Geometry check sheet. Reference: the model listing, model coordinates, mm. Face numbers are marked on the shaded views. A direction names the side the tool comes from. Round coordinates to 2 decimals unless told otherwise and drop trailing zeros. Write each loop counter-clockwise with the first axis right and the second up, starting at its lowest first coordinate (ties: lowest second). Pieces come first, ordered by that corner, then holes. Notation, with made-up numbers: M -22,13 L 37,13 A35 cw 37,50 Z; hole C 72.25,-29.5 d8. An arc over 180 degrees is marked long. Put each result on its own line as item: value. Start each with the question number.
(1) Section check C-C on y = 12. Record the cut outline in (x, z).
(2) Material ranges on probe 1 along Y at (x, z) = (6.5, 0); probe 2 along Z at (x, y) = (6, 0); probe 3 along Y at (x, z) = (20, -26), recorded low to high.
(3) Gauge pin test, flat ends, axial feed: pin 1 (10 mm diameter, centred on x = -12.5, z = -13, fed in from -Y); pin 2 (8 mm diameter, centred on x = -10.27, y = 0, fed in from +Z); pin 3 (12 mm diameter, centred on x = 13.5, z = 7.5, fed in from -Y); pin 4 (8 mm diameter, centred on y = 17, z = -15.5, fed in from +X). Record the tip position at first contact, or that the pin passes through.
(4) Section check D-D on x = 3. Record the cut outline in (y, z).
(5) Section check A-A on x = 20. Record the cut outline in (y, z).
(6) Section check B-B on z = -12.5. Record the cut outline in (x, y).
(7) Tool access check on the marked faces 1, 2 and 3. Record the directions out of +Z, -Z, +X, -X, +Y, -Y that give a thin tool (end or side, any length) a straight path to the whole face; none if there is none.
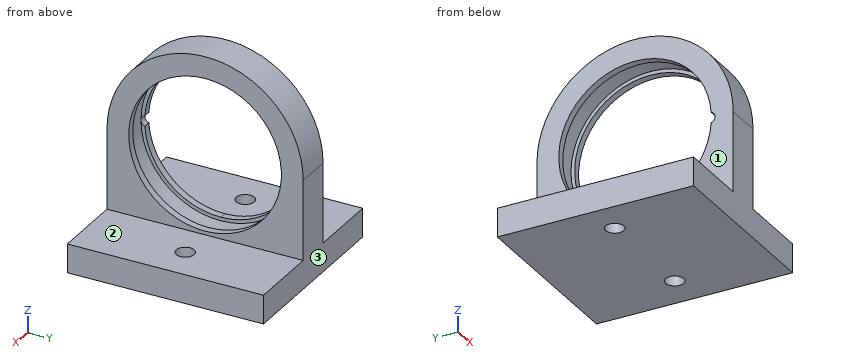
Autodesk Inventor part; units mm, degrees
ref_plane "Work Plane8" through (0, 0, 0) normal (0, -1, 0) x (1, 0, 0)
ref_plane "YZ Plane" through (0, 0, 0) normal (1, 0, 0) x (0, 1, 0)
ref_plane "XZ Plane" through (0, 0, 0) normal (0, 1, 0) x (-1, 0, 0)
sketch "Sketch15" plane through (0, 0, 0) normal (1, 0, 0) x (0, 1, 0)
  circle A0 centre (0, 0) radius 22
  circle A1 centre (0, 0) radius 27
  line L0 (27, 0) -> (27, -29.9149)
  line L1 (27, -29.9149) -> (-27, -29.9149)
  line L2 (-27, -29.9149) -> (-27, 0)
  dimension "d51" = 44
  dimension "d52" = 54
extrude "Extrusion11" add sketch "Sketch15" along normal blind 10
sketch "Sketch16" plane through (10, 0, 0) normal (1, 0, 0) x (0, 0, -1)
  line L0 (29.9149, -27) -> (29.9149, 27)
  circle A0 centre (0, 0) radius 22
  line L1 (29.9149, 27) -> (22, 27)
  line L2 (22, 27) -> (22, 0)
  line L3 (22, 0) -> (29.9149, 0)
  line L4 (29.9149, 0) -> (29.9149, 27)
  line L5 (0, -27) -> (29.9149, -27)
  line L6 (22, 0) -> (29.9149, 0)
  line L7 (29.9149, 0) -> (29.9149, -27)
  line L8 (29.9149, -27) -> (22, -27)
  line L9 (22, -27) -> (22, 0)
extrude "Extrusion12" add sketch "Sketch16" along normal blind 20 contours L5 L9 L3 L0 | L3 L2 L1 L0
sketch "Sketch17" plane through (0, 0, 0) normal (-1, 0, 0) x (0, 0, 1)
  line L0 (-29.9149, -27) -> (-29.9149, 27)
  circle A0 centre (0, 0) radius 22
  line L1 (-29.9149, 27) -> (-22, 27)
  line L2 (-22, 27) -> (-22, 0)
  line L3 (-22, 0) -> (-29.9149, 0)
  line L4 (-29.9149, 0) -> (-29.9149, 27)
  line L5 (0, -27) -> (-29.9149, -27)
  line L6 (-22, 0) -> (-29.9149, 0)
  line L7 (-29.9149, 0) -> (-29.9149, -27)
  line L8 (-29.9149, -27) -> (-22, -27)
  line L9 (-22, -27) -> (-22, 0)
extrude "Extrusion13" add sketch "Sketch17" along normal blind 20 contours L0 L3 L9 L5 | L0 L1 L2 L3
ref_plane "Work Plane8" through (0, 0, 0) normal (0, -1, 0) x (1, 0, 0)
sketch "Sketch18" plane through (0, 0, 0) normal (0, -1, 0) x (1, 0, 0)
  line L0 (0, 0) -> (0, -22)
  line L1 (0, -22) -> (2, -22)
  line L2 (10, -22) -> (0, -22)
  line L3 (0, -22) -> (0, -21)
  line L4 (0, -21) -> (2, -21)
  line L5 (2, -22) -> (2, -21)
  line L6 (10, -22) -> (8, -22)
  line L7 (8, -22) -> (8, -21)
  line L8 (8, -21) -> (10, -21)
  line L9 (10, -21) -> (10, -22)
  line L10 (-30, 0) -> (40, 0)
  dimension "d59" = 2
  dimension "d60" = 1
  dimension "d61" = 2
  dimension "d62" = 1
revolve "Revolution3" add sketch "Sketch18" angle 360 about axis through (-10, 0, 0) along (1, 0, 0)
sketch "Sketch19" plane through (10, -27, -22) normal (0, 0, 1) x (1, 0, 0)
  line L0 (20, 54) -> (20, 0)
  line L1 (20, 27) -> (10, 27)
  line L2 (-30.2682, 27) -> (-20.2682, 27)
  circle A0 centre (-20.2682, 27) radius 2.5
  circle A1 centre (10, 27) radius 2.5
  point P0 (-10, 27)
  dimension "d64" = 10
  dimension "d65" = 10
  dimension "d66" = 5
  dimension "d67" = 5
extrude "Extrusion14" cut sketch "Sketch19" against normal blind 20
sketch "Sketch20" plane through (2, 0, 0) normal (1, 0, 0) x (0, 0, -1)
  circle A0 centre (0, 0) radius 22
  line L0 (0, -22) -> (0, -20.5)
  circle A1 centre (0, -20.5) radius 1.5
  dimension "d71" = 1.5
extrude "Extrusion15" cut sketch "Sketch20" against normal blind 20 contours A1
properties part number "antenna_rad_outter"
Answers follow:
1. outline: M -20,-29.91 L 30,-29.91 L 30,-22 L 10,-22 L 10,-17.23 L 8,-17.23 L 8,-18.44 L 2,-18.44 L 2,-17.23 L 0,-17.23 L 0,-22 L -20,-22 Z; M 0,17.23 L 2,17.23 L 2,18.44 L 8,18.44 L 8,17.23 L 10,17.23 L 10,24.19 L 0,24.19 Z
2. probe 1: y = -27 to -22, 22 to 27
2. probe 2: z = -29.91 to -22, 22 to 27
2. probe 3: y = -27 to -2.5, 2.5 to 27
3. pin 1: passes through
3. pin 2: stops at z = -22
3. pin 3: stops at y = -26.87
3. pin 4: stops at x = 10
4. outline: M -27,-29.91 L 27,-29.91 L 27,0 A27 ccw -27,0 Z; hole C 0,0 d44
5. outline: M -27,-29.91 L -2.5,-29.91 L -2.5,-22 L -27,-22 Z; M 2.5,-29.91 L 27,-29.91 L 27,-22 L 2.5,-22 Z
6. outline: M 0,-27 L 10,-27 L 10,-16.87 L 8,-16.87 L 8,-18.1 L 2,-18.1 L 2,-16.87 L 0,-16.87 Z; M 0,16.87 L 2,16.87 L 2,18.1 L 8,18.1 L 8,16.87 L 10,16.87 L 10,27 L 0,27 Z
7. face 1: +Z, -X, +Y, -Y
7. face 2: +Z, +X, +Y, -Y
7. face 3: +Z, -Z, +X, -X, +Y
